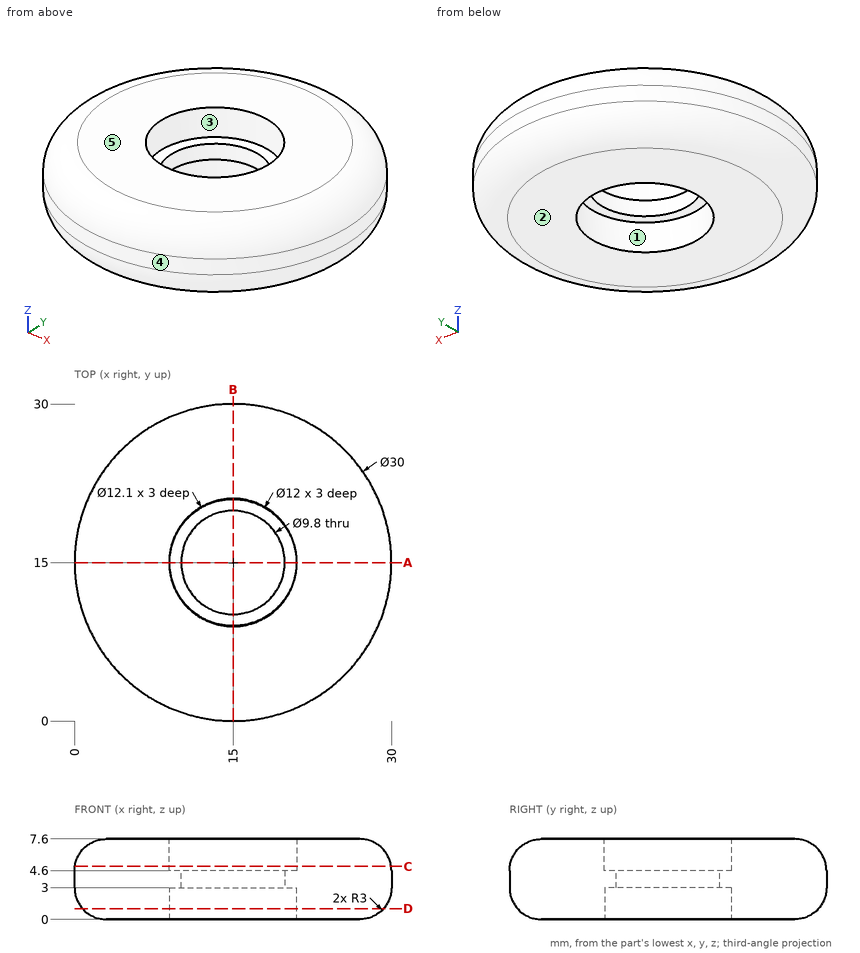
Check sheet for the drawn part. Datum: minimum x, y, z corner. Units: mm. A direction names the side the tool comes from. Give positions to 0.01 mm unless a question says otherwise; leave off trailing zeros. Loops run counter-clockwise (first coordinate to the right, second up) from the corner with the lowest first, then second, coordinate; pieces in that order, holes last.
1) Sectioned sample at A-A, the plane y = 15. Enter the section's corners in (x, z).
2) Draft check along Y on the marked faces 3, 4 and 5. Enter one of: pulls with the +Y half, pulls with the -Y half, needs draft (parallel to the pull), parting line crosses it, or undercut.
3) Depth check by flat-ended pin: pin 1 Ø11 at (x, y) = (15, 15) entering from -Z; pin 2 Ø4 at (x, z) = (12, 5) entering from -Y; pin 3 Ø3 at (y, z) = (22, 1) entering from -X. Enter the tip coordinate at first touch or a pass-through.
4) Sectioned sample at C-C, the plane z = 5. Enter the section's corners in (x, y), then the cut area to 3 significant figures.
5) Thickness scan on line 1 along Y through (x, z) = (15, 4.2); line 2 along Y through (x, z) = (14.5, 1); line 3 along X through (y, z) = (19.5, 2.75). Record the ranges inside material, lowest first.
6) Sectioned sample at D-D, the plane z = 1. Enter the section's corners in (x, y), then the cut area to 3 significant figures.
7) Set-up check for the marked faces 1 and 2: record each of +Z, -Z, +X, -X, +Y, -Y from which the full face is reachable in a straight line by a thin tool's end or side.
Answers:
1. outline: (0, 3) arc R3 ccw to (3, 0) - (9, 0) - (9, 3) - (10.1, 3) - (10.1, 4.6) - (8.95, 4.6) - (8.95, 7.6) - (3, 7.6) arc R3 ccw to (0, 4.6) - close; (19.9, 3) - (21, 3) - (21, 0) - (27, 0) arc R3 ccw to (30, 3) - (30, 4.6) arc R3 ccw to (27, 7.6) - (21.05, 7.6) - (21.05, 4.6) - (19.9, 4.6) - close
2. face 3: undercut
2. face 4: parting line crosses it
2. face 5: needs draft
3. pin 1: stops at z = 3
3. pin 2: stops at y = 0.04
3. pin 3: stops at x = 1.39
4. outline: circle Ø29.95 at (15, 15); hole circle Ø12.1 at (15, 15)
4. area: 589 mm2
5. line 1: y = 0 to 10.1, 19.9 to 30
5. line 2: y = 0.77 to 9.02, 20.98 to 29.23
5. line 3: x = 0.7 to 11.03, 18.97 to 29.3
6. outline: circle Ø28.47 at (15, 15); hole circle Ø12 at (15, 15)
6. area: 524 mm2
7. face 1: -Z
7. face 2: -Z, +X, -X, +Y, -Y
